Input: dimensioned drawing with shaded views. Units: mm. Origin: part minimum x, y, z. A direction names the side the tool comes from. Round coordinates to 2 decimals unless told otherwise and drop trailing zeros. Order: outer loops, then holes, each group sorted by start corner. A loop starts at its lowest first (then second) coordinate and runs counter-clockwise, first axis right, second up. Notation, with made-up numbers: (17.5, 15) -> (29.5, 15) arc R24 cw to (29.5, 42) -> close; hole circle Ø5 at (81, 9). An arc over 180 degrees is marked (long way). Use a Markdown table: item, result. Add a question column.
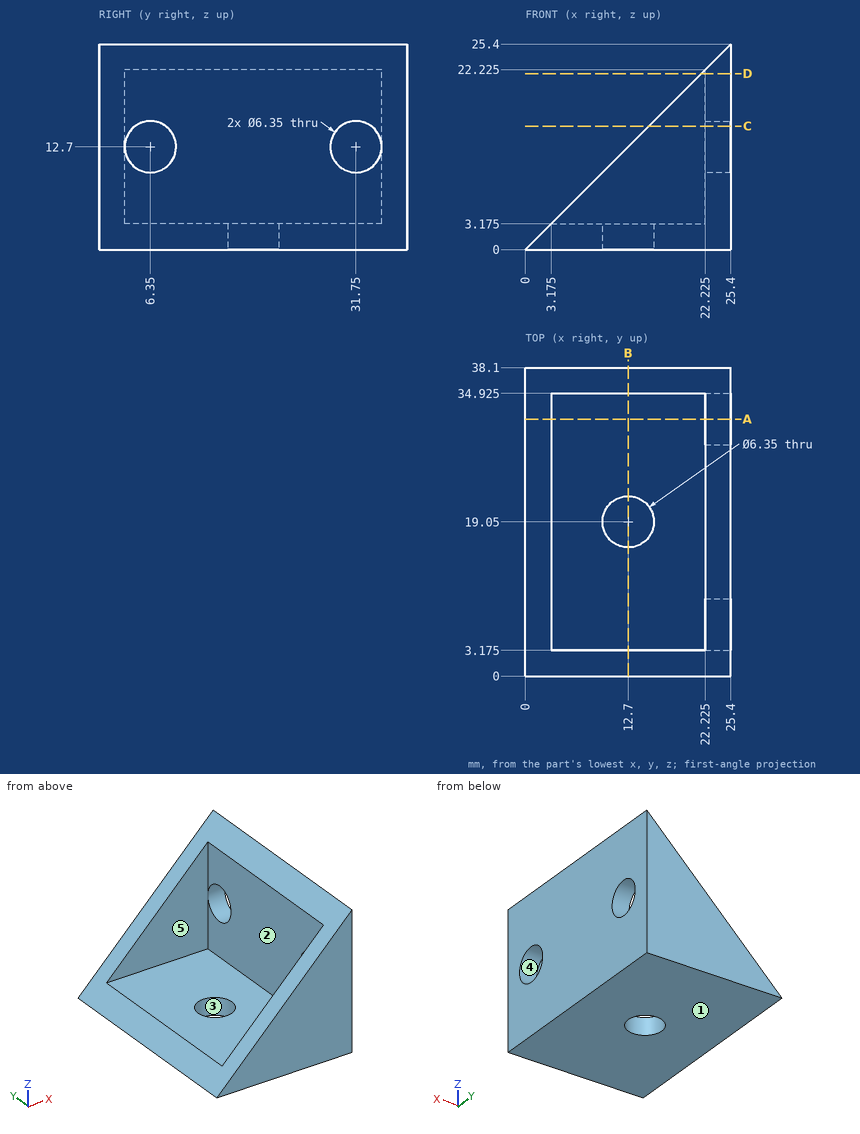
1) Section D-D on z = 21.75. Output: boundary loops of the cut face in (x, y) (3 decimals), then the cut area to 3 significant figures.
2) Reachability of the marked faces 4 and 5 from +Z, -Z, +X, -X, +Y, -Y: full face, straight path, thin tool, end or side. Return the list, or none.
3) First-contact query: pin 1 Ø12 at (x, y) = (5, 14) entering from +Z (3 decimals); pin 2 Ø8 at (x, y) = (20.5, 29) entering from +Z; pin 3 Ø5.5 at (y, z) = (18.5, 15) entering from -X (3 decimals). Flat tips, straight axial feed; report the tip coordinate or a pass-through.
4) Section A-A on y = 31.75. Output: boundary loops of the cut face in (x, z) (3 decimals), then the cut area to 3 significant figures.
5) Line query: probe 1 along Y at (x, z) = (24.3, 12.7) (3 decimals); probe 2 along Y at (x, z) = (20.5, 13.25) (3 decimals); probe 3 along Z at (x, y) = (13.75, 23.5) (3 decimals). Output: solid intervals per line, ascending. Write a range as from..to.
6) Section C-C on z = 15.25. Output: boundary loops of the cut face in (x, y) (3 decimals), then the cut area to 3 significant figures.
7) Draft query along X for the marked faces 1, 2 and 3. Return one class per face: pulls with the +X half, pulls with the -X half, needs draft (parallel to the pull), parting line crosses it, or undercut.
8) Section B-B on x = 12.7. Output: boundary loops of the cut face in (y, z) (3 decimals), then the cut area to 3 significant figures.
Conclusion:
| question | item | result |
|---|---|---|
| 1 | outline | (21.75, 0) -> (25.4, 0) -> (25.4, 38.1) -> (21.75, 38.1) -> (21.75, 34.925) -> (22.225, 34.925) -> (22.225, 3.175) -> (21.75, 3.175) -> close |
| 1 | area | 124 mm^2 |
| 2 | face 4 | +X, -X |
| 2 | face 5 | +Z, -X |
| 3 | pin 1 | stops at z = 3.175 |
| 3 | pin 2 | stops at z = 24.5 |
| 3 | pin 3 | stops at x = 22.225 |
| 4 | outline | (0, 0) -> (25.4, 0) -> (25.4, 9.525) -> (22.225, 9.525) -> (22.225, 3.175) -> (3.175, 3.175) -> close; (22.225, 15.875) -> (25.4, 15.875) -> (25.4, 25.4) -> (22.225, 22.225) -> close |
| 4 | area | 121 mm^2 |
| 5 | probe 1 | y = 0..3.175, 9.525..28.575, 34.925..38.1 |
| 5 | probe 2 | y = 0..3.175, 34.925..38.1 |
| 5 | probe 3 | z = 0..3.175 |
| 6 | outline | (15.25, 0) -> (25.4, 0) -> (25.4, 4.458) -> (22.225, 4.458) -> (22.225, 3.175) -> (15.25, 3.175) -> close; (15.25, 34.925) -> (22.225, 34.925) -> (22.225, 33.642) -> (25.4, 33.642) -> (25.4, 38.1) -> (15.25, 38.1) -> close; (22.225, 8.242) -> (25.4, 8.242) -> (25.4, 29.858) -> (22.225, 29.858) -> close |
| 6 | area | 141 mm^2 |
| 7 | face 1 | needs draft |
| 7 | face 2 | pulls with the -X half |
| 7 | face 3 | undercut |
| 8 | outline | (0, 0) -> (15.875, 0) -> (15.875, 3.175) -> (3.175, 3.175) -> (3.175, 12.7) -> (0, 12.7) -> close; (22.225, 0) -> (38.1, 0) -> (38.1, 12.7) -> (34.925, 12.7) -> (34.925, 3.175) -> (22.225, 3.175) -> close |
| 8 | area | 161 mm^2 |
